The model under review builds one solid part; all positions refer to its coordinate system, in mm. Coordinates: 2 decimals unless noted, no trailing zeros. Write each loop counter-clockwise with the first axis right and the second up, starting at its lowest first coordinate (ties: lowest second). Pieces come first, ordered by that corner, then holes. Notation, with made-up numbers: (-12, 49.25) - (26, 49.25) arc R29 cw to (26, 71.25) - close; hole circle Ø8 at (64.25, 27.25). An arc over 180 degrees is marked (long way). Use one line per item in the form item = value. Start each with the question number.
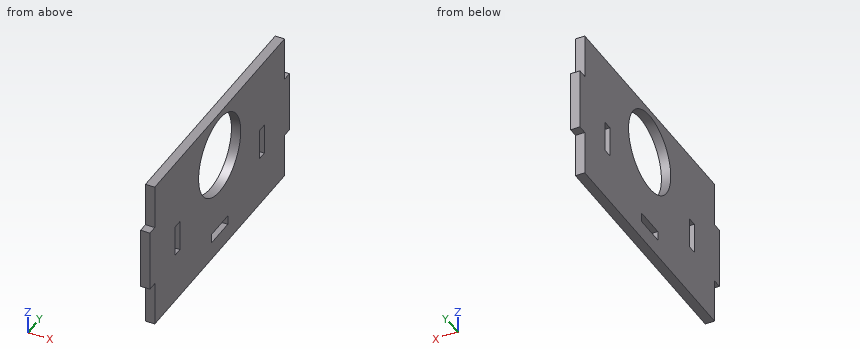
Solid Edge part; units mm, degrees
sketch "Sketch1" plane through (0, 0, 0) normal (1, 0, 0) x (0, 1, 0)
  line L0 (-5, 8.8) -> (5, 8.8)
  line L1 (5, 8.8) -> (5, 5.8)
  line L2 (5, 5.8) -> (-5, 5.8)
  line L3 (-5, 5.8) -> (-5, 8.8)
  line L4 (24.5, 26.3) -> (24.5, 16.3)
  line L5 (24.5, 16.3) -> (27.5, 16.3)
  line L6 (27.5, 16.3) -> (27.5, 26.3)
  line L7 (27.5, 26.3) -> (24.5, 26.3)
  line L8 (-24.5, 26.3) -> (-24.5, 16.3)
  line L9 (-24.5, 16.3) -> (-27.5, 16.3)
  line L10 (-27.5, 16.3) -> (-27.5, 26.3)
  line L11 (-27.5, 26.3) -> (-24.5, 26.3)
  circle A0 centre (0, 33.8) radius 13
  line L12 (-40, 48.8) -> (-40, 34.4)
  line L13 (-40, 34.4) -> (-43, 34.4)
  line L14 (-43, 34.4) -> (-43, 14.4)
  line L15 (-43, 14.4) -> (-40, 14.4)
  line L16 (-40, 14.4) -> (-40, 0)
  line L17 (-40, 0) -> (40, 0)
  line L18 (40, 0) -> (40, 14.4)
  line L19 (40, 14.4) -> (43, 14.4)
  line L20 (43, 14.4) -> (43, 34.4)
  line L21 (43, 34.4) -> (40, 34.4)
  line L22 (40, 34.4) -> (40, 48.8)
  line L23 (40, 48.8) -> (-40, 48.8)
  dimension "D1" = 43
  dimension "D2" = 40
  dimension "D3" = 5
  dimension "D4" = 40
  dimension "D5" = 40
extrude "Protrusion1" add sketch "Sketch1" against normal blind 3
properties material "Acier"
1. For P1, Ø0.9, axis at x = -1, z = 8.5, coming from the -Y side; P2, Ø0.9, axis at x = -2, z = 5, coming from the +Y side; P3, Ø1.5, axis at x = -2, y = 42, coming from the -Z side, all flat-tipped, find the tip position at first contact; note any pin that passes through.
2. For L1, parallel to Z at x = -1.25, y = 0; L2, parallel to Z at x = -2.9, y = -26; L3, parallel to Z at x = -0.8, y = 3.5, list the stretches that pass through material, from the lowest coordinate up.
3. Take a section at D-D (z = 32). State the section outline as (x, y) points, plus the area to 3 significant figures.
4. Take a section at B-B (x = -1.25). State the section outline as (y, z) points.
5. Take a section at C-C (y = 0). State the section outline as (x, z) points.
6. Take a section at A-A (z = 18.5). State the section outline as (x, y) points, plus the area to 3 significant figures.
Returned:
q1.P1 = -40
q1.P2 = 40
q1.P3 = 14.4
q2.L1 = 0 to 5.8, 8.8 to 20.8, 46.8 to 48.8
q2.L2 = 0 to 16.3, 26.3 to 48.8
q2.L3 = 0 to 5.8, 8.8 to 21.28, 46.32 to 48.8
q3.outline = (-3, -43) - (0, -43) - (0, -12.87) - (-3, -12.87) - close; (-3, 12.87) - (0, 12.87) - (0, 43) - (-3, 43) - close
q3.area = 181 mm²
q4.outline = (-43, 14.4) - (-40, 14.4) - (-40, 0) - (40, 0) - (40, 14.4) - (43, 14.4) - (43, 34.4) - (40, 34.4) - (40, 48.8) - (-40, 48.8) - (-40, 34.4) - (-43, 34.4) - close; hole (-27.5, 16.3) - (-24.5, 16.3) - (-24.5, 26.3) - (-27.5, 26.3) - close; hole circle Ø26 at (0, 33.8); hole (-5, 5.8) - (5, 5.8) - (5, 8.8) - (-5, 8.8) - close; hole (24.5, 16.3) - (27.5, 16.3) - (27.5, 26.3) - (24.5, 26.3) - close
q5.outline = (-3, 0) - (0, 0) - (0, 5.8) - (-3, 5.8) - close; (-3, 8.8) - (0, 8.8) - (0, 20.8) - (-3, 20.8) - close; (-3, 46.8) - (0, 46.8) - (0, 48.8) - (-3, 48.8) - close
q6.outline = (-3, -43) - (0, -43) - (0, -27.5) - (-3, -27.5) - close; (-3, -24.5) - (0, -24.5) - (0, 24.5) - (-3, 24.5) - close; (-3, 27.5) - (0, 27.5) - (0, 43) - (-3, 43) - close
q6.area = 240 mm²
